Work out the finished part from the listing and answer in its coordinate system (mm). A direction names the side the tool comes from. Give positions to 0.01 mm unless a question says otherwise; leave off trailing zeros. Write each loop counter-clockwise with the first axis right and the second up, starting at its lowest first coordinate (ties: lowest second). Pieces come first, ordered by that corner, then holes.
1) A tool of negligible diameter and unlimited length cuts with its end or side. For faces 5 (the face through (-472.6, -3, 36)), 6 (the face through (254, -63.5, -138)), 7 (the face through (-242, 145, -38.1)), 8 (the face through (228.6, -76, -138)), 9 (the face through (254, 215.9, -138)), from which of +Z, -Z, +X, -X, +Y, -Y can it reach the whole face along a straight path? Write none if from no direction.
2) Find section A-A (y = 139.7). Determine the outline of the cut face in (x, z), plus the area to 3 significant figures.
3) Given pin 1 Ø3 at (x, y) = (-297.5, 79) entering from -Z; pin 2 Ø12.5 at (y, z) = (-71, -126) entering from +X; pin 3 Ø5 at (y, z) = (139, 181) entering from -X, each flat-ended and moving along its own axis, determine where each tip first touches the part or whether it passes through.
4) Straight lines are drawn through the part: probe 1 along Y at (x, z) = (-254, -21); probe 2 along Y at (x, z) = (-254, 5); probe 3 along Z at (x, y) = (-134, 181). For each, find the intervals that lie inside material, in ascending order.
5) Find section C-C (x = -157.5). Determine the outline of the cut face in (y, z), plus the area to 3 significant figures.
6) Determine the mould class of faces 1 (the face through (228.6, 76, -138)), 2 (the face through (-437.886, 3.815, -25.756)), 3 (the face through (254, 203, -228.6)), 4 (the face through (192.93, -20, 220.54)) for opening direction X: pulls with the +X half, pulls with the -X half, needs draft (parallel to the pull), parting line crosses it, or undercut.
7) Find section D-D (y = -34). Determine the outline of the cut face in (x, z).
8) Find section B-B (z = -61). Determine the outline of the cut face in (x, y), plus the area to 3 significant figures.
```python
from build123d import *

# Parameters (mm, degrees)
SKETCH1_W                = 965.2
SKETCH1_H                = 508
BOSS_EXTRUDE1_DEPTH      = 50.8
SKETCH3_W                = 50.8
SKETCH3_H                = 25.4
BOSS_EXTRUDE2_DEPTH      = 177.8
CUT_EXTRUDE2_DEPTH       = 592.334693723
CUT_EXTRUDE2_DEPTH_BACK  = 592.334693723
SKETCH4_R                = 12.7
BOSS_EXTRUDE3_DEPTH      = 254
BOSS_EXTRUDE3_DEPTH_BACK = 254
BOSS_EXTRUDE4_DEPTH      = 12.7
BOSS_EXTRUDE5_START      = -508
BOSS_EXTRUDE5_DEPTH      = 12.7
CUT_EXTRUDE3_DEPTH       = 592.556393084
CUT_EXTRUDE3_DEPTH_BACK  = 592.556393084
SKETCH2_R                = 12.7
CUT_EXTRUDE4_START       = -50.8
SKETCH12_R               = 25.4
SKETCH12_R_2             = 12.7
CUT_EXTRUDE4_DEPTH       = 12.7
SKETCH13_R               = 12.7
CUT_EXTRUDE5_DEPTH       = 25.4
CUT_EXTRUDE6_START       = -2.7
SKETCH14_R               = 25.4
SKETCH14_R_2             = 12.7
CUT_EXTRUDE6_DEPTH       = 12.7
CUT_EXTRUDE7_DEPTH       = 10
CUT_EXTRUDE7_DEPTH_BACK  = 592.556393084
SKETCH15_R               = 12.7
SKETCH2_4_R              = 12.7
BOSS_EXTRUDE6_DEPTH      = 150
CUT_EXTRUDE8_REACH       = 714.022
SKETCH16_R               = 4.5
CUT_EXTRUDE9_REACH       = 823.718
SKETCH17_W               = 300
SKETCH17_H               = 450


with BuildPart() as part:
    # Sketch1 → Boss-Extrude1 (new body)
    with BuildSketch(Plane.XY):
        Rectangle(SKETCH1_W, SKETCH1_H)
    extrude(amount=-BOSS_EXTRUDE1_DEPTH)

    # Sketch3 → Boss-Extrude2 (add)
    with BuildSketch(Plane(origin=(0, 0, -50.8), x_dir=(-1, 0, 0), z_dir=(0, 0, -1))):
        with Locations((-254, 203.2)):
            Rectangle(SKETCH3_W, SKETCH3_H)
        with Locations((-254, 76.2)):
            Rectangle(SKETCH3_W, SKETCH3_H)
        with Locations((-254, -76.2)):
            Rectangle(SKETCH3_W, SKETCH3_H)
        with Locations((-254, -203.2)):
            Rectangle(SKETCH3_W, SKETCH3_H)
    extrude(amount=BOSS_EXTRUDE2_DEPTH)

    # Sketch4 → Cut-Extrude2 (cut, two sides: drawn at the far end of the back side and taken through both)
    with BuildSketch(Plane(origin=(0, 0, 0), x_dir=(1, 0, 0), z_dir=(0, 1, 0)).offset(-CUT_EXTRUDE2_DEPTH_BACK)):
        with Locations(Location((254, 190.5, 0), (0, 0, 270))):
            Circle(SKETCH4_R)
    extrude(amount=CUT_EXTRUDE2_DEPTH + CUT_EXTRUDE2_DEPTH_BACK, mode=Mode.SUBTRACT)

    # Sketch10 → Boss-Extrude3 (add, two sides: drawn at the far end of the back side and taken through both)
    with BuildSketch(Plane(origin=(0, 0, 0), x_dir=(1, 0, 0), z_dir=(0, 1, 0)).offset(-BOSS_EXTRUDE3_DEPTH_BACK)):
        Polygon((482.6, 0), (-482.6, 0), (-482.6, -66.924314291), (-176.649889789, -229.172874046), (0, -229.172874046), (176.649889789, -229.172874046), (482.6, -66.924314291), align=None)
        Polygon((-472.6, -60.908279697), (-472.6, -10), (472.6, -10), (472.6, -60.908279697), (174.162404273, -219.172874046), (0, -219.172874046), (-174.162404273, -219.172874046), align=None, mode=Mode.SUBTRACT)
    extrude(amount=BOSS_EXTRUDE3_DEPTH + BOSS_EXTRUDE3_DEPTH_BACK)

    # Sketch11 → Boss-Extrude4 (add)
    with BuildSketch(Plane.XZ.offset(254)):
        Polygon((-472.6, 10), (-472.6, 60.908279697), (-174.162404273, 219.172874046), (174.162404273, 219.172874046), (472.6, 60.908279697), (472.6, 10), align=None)
    extrude(amount=-BOSS_EXTRUDE4_DEPTH)

    # Sketch11<2> → Boss-Extrude5 (add)
    with BuildSketch(Plane.XZ.offset(254).offset(BOSS_EXTRUDE5_START)):
        Polygon((-472.6, 10), (-472.6, 60.908279697), (-174.162404273, 219.172874046), (174.162404273, 219.172874046), (472.6, 60.908279697), (472.6, 10), align=None)
    extrude(amount=BOSS_EXTRUDE5_DEPTH)

    # Sketch2 → Cut-Extrude3 (cut, two sides: drawn at the far end of the back side and taken through both)
    with BuildSketch(Plane.XY.offset(-CUT_EXTRUDE3_DEPTH_BACK)):
        with Locations((-450, 0)):
            Circle(SKETCH2_R)
    extrude(amount=CUT_EXTRUDE3_DEPTH + CUT_EXTRUDE3_DEPTH_BACK, mode=Mode.SUBTRACT)

    # Sketch12 → Cut-Extrude4 (cut)
    # profile 1 of 2: a face of its own
    with BuildSketch(Plane.XY.offset(CUT_EXTRUDE4_START)):
        with Locations(Location((-254, 139.7, 0), (0, 0, 180))):
            Circle(SKETCH12_R)
        with Locations(Location((-254, 139.7, 0), (0, 0, 180))):
            Circle(SKETCH12_R_2, mode=Mode.SUBTRACT)
    # profile 2 of 2: a face of its own
    with BuildSketch(Plane.XY.offset(CUT_EXTRUDE4_START)):
        with Locations(Location((-254, -139.7, 0), (0, 0, 180))):
            Circle(SKETCH12_R)
        with Locations(Location((-254, -139.7, 0), (0, 0, 180))):
            Circle(SKETCH12_R_2, mode=Mode.SUBTRACT)
    extrude(amount=CUT_EXTRUDE4_DEPTH, mode=Mode.SUBTRACT)

    # Sketch13 → Cut-Extrude5 (cut)
    with BuildSketch(Plane(origin=(0, 0, -50.8), x_dir=(-1, 0, 0), z_dir=(0, 0, -1))):
        with Locations((254, 139.7)):
            Circle(SKETCH13_R)
        with Locations((254, -139.7)):
            Circle(SKETCH13_R)
    extrude(amount=-CUT_EXTRUDE5_DEPTH, mode=Mode.SUBTRACT)

    # Sketch14 → Cut-Extrude6 (cut)
    # profile 1 of 2: a face of its own
    with BuildSketch(Plane.XY.offset(CUT_EXTRUDE6_START)):
        with Locations(Location((-254, 139.7, 0), (0, 0, 180))):
            Circle(SKETCH14_R)
        with Locations(Location((-254, 139.7, 0), (0, 0, 180))):
            Circle(SKETCH14_R_2, mode=Mode.SUBTRACT)
    # profile 2 of 2: a face of its own
    with BuildSketch(Plane.XY.offset(CUT_EXTRUDE6_START)):
        with Locations(Location((-254, -139.7, 0), (0, 0, 180))):
            Circle(SKETCH14_R)
        with Locations(Location((-254, -139.7, 0), (0, 0, 180))):
            Circle(SKETCH14_R_2, mode=Mode.SUBTRACT)
    extrude(amount=CUT_EXTRUDE6_DEPTH, mode=Mode.SUBTRACT)

    # Sketch15 → Cut-Extrude7 (cut, two sides: drawn at the far end of the back side and taken through both)
    with BuildSketch(Plane.XY.offset(-CUT_EXTRUDE7_DEPTH_BACK)):
        with Locations(Location((-254, -139.7, 0), (0, 0, 180))):
            Circle(SKETCH15_R)
        with Locations(Location((-254, 139.7, 0), (0, 0, 180))):
            Circle(SKETCH15_R)
    extrude(amount=CUT_EXTRUDE7_DEPTH + CUT_EXTRUDE7_DEPTH_BACK, mode=Mode.SUBTRACT)

    # Sketch2<4> → Boss-Extrude6 (add)
    with BuildSketch(Plane.XY):
        with Locations((-450, 0)):
            Circle(SKETCH2_4_R)
    extrude(amount=BOSS_EXTRUDE6_DEPTH)

    # Sketch16 → Cut-Extrude8 (cut, up to next)
    with BuildSketch(Plane.XY.offset(229.172874046), mode=Mode.PRIVATE) as cut_extrude8_sk1:
        with Locations((-66, 0)):
            Circle(SKETCH16_R)
    cut_extrude8_tool1 = extrude(cut_extrude8_sk1.sketch, amount=-CUT_EXTRUDE8_REACH, mode=Mode.PRIVATE) & part.part
    # Sketch16 → Cut-Extrude8 (cut, up to next)
    with BuildSketch(Plane.XY.offset(229.172874046), mode=Mode.PRIVATE) as cut_extrude8_sk2:
        with Locations((0, 66)):
            Circle(SKETCH16_R)
    cut_extrude8_tool2 = extrude(cut_extrude8_sk2.sketch, amount=-CUT_EXTRUDE8_REACH, mode=Mode.PRIVATE) & part.part
    # Sketch16 → Cut-Extrude8 (cut, up to next)
    with BuildSketch(Plane.XY.offset(229.172874046), mode=Mode.PRIVATE) as cut_extrude8_sk3:
        with Locations((66, 0)):
            Circle(SKETCH16_R)
    cut_extrude8_tool3 = extrude(cut_extrude8_sk3.sketch, amount=-CUT_EXTRUDE8_REACH, mode=Mode.PRIVATE) & part.part
    # Sketch16 → Cut-Extrude8 (cut, up to next)
    with BuildSketch(Plane.XY.offset(229.172874046), mode=Mode.PRIVATE) as cut_extrude8_sk4:
        with Locations((0, -66)):
            Circle(SKETCH16_R)
    cut_extrude8_tool4 = extrude(cut_extrude8_sk4.sketch, amount=-CUT_EXTRUDE8_REACH, mode=Mode.PRIVATE) & part.part
    add(cut_extrude8_tool1.solids().sort_by_distance((-66, 0, 229.172874))[0], mode=Mode.SUBTRACT)
    add(cut_extrude8_tool2.solids().sort_by_distance((0, 66, 229.172874))[0], mode=Mode.SUBTRACT)
    add(cut_extrude8_tool3.solids().sort_by_distance((66, 0, 229.172874))[0], mode=Mode.SUBTRACT)
    add(cut_extrude8_tool4.solids().sort_by_distance((0, -66, 229.172874))[0], mode=Mode.SUBTRACT)

    # Sketch17 → Cut-Extrude9 (cut, up to next)
    with BuildSketch(Plane(origin=(133.630964067, 0, 251.986262594), x_dir=(0.8834593660439969, 0, -0.4685077892086097), z_dir=(0.4685077892086097, 0, 0.8834593660439969)), mode=Mode.PRIVATE) as cut_extrude9_sk1:
        with Locations((217.872449791, 0)):
            Rectangle(SKETCH17_W, SKETCH17_H)
    cut_extrude9_tool1 = extrude(cut_extrude9_sk1.sketch, amount=-CUT_EXTRUDE9_REACH, mode=Mode.PRIVATE) & part.part
    add(cut_extrude9_tool1.solids().sort_by_distance((326.11242, 0, 149.911323))[0], mode=Mode.SUBTRACT)


solid = part.part
```
Results:
1. face 5: none
1. face 6: -Z, +X, -X
1. face 7: -Z
1. face 8: -Z, -X, +Y, -Y
1. face 9: -Z, +X, -X, +Y
2. outline: (-482.6, -50.8) - (-279.4, -50.8) - (-279.4, -38.1) - (-266.7, -38.1) - (-266.7, -2.7) - (-279.4, -2.7) - (-279.4, 10) - (-472.6, 10) - (-472.6, 60.91) - (-174.16, 219.17) - (174.16, 219.17) - (188.91, 211.35) - (193.59, 220.19) - (176.65, 229.17) - (-176.65, 229.17) - (-482.6, 66.92) - close; (-241.3, -38.1) - (-228.6, -38.1) - (-228.6, -50.8) - (482.6, -50.8) - (482.6, 66.92) - (458.63, 79.64) - (453.95, 70.8) - (472.6, 60.91) - (472.6, 10) - (-228.6, 10) - (-228.6, -2.7) - (-241.3, -2.7) - close
2. area: 64,900 mm2
3. pin 1: stops at z = -50.8
3. pin 2: stops at x = 279.4
3. pin 3: stops at x = -272.2
4. probe 1: y = -254 to -152.4, -127 to 127, 152.4 to 254
4. probe 2: y = -254 to -165.1, -114.3 to 114.3, 165.1 to 254
4. probe 3: z = -50.8 to 10, 219.17 to 229.17
5. outline: (-254, -50.8) - (254, -50.8) - (254, 229.17) - (-254, 229.17) - close; hole (-241.3, 10) - (241.3, 10) - (241.3, 219.17) - (-241.3, 219.17) - close
5. area: 41,300 mm2
6. face 1: pulls with the -X half
6. face 2: undercut
6. face 3: needs draft
6. face 4: pulls with the +X half
7. outline: (-482.6, -50.8) - (482.6, -50.8) - (482.6, 66.92) - (458.63, 79.64) - (453.95, 70.8) - (472.6, 60.91) - (472.6, 10) - (-472.6, 10) - (-472.6, 60.91) - (-174.16, 219.17) - (174.16, 219.17) - (188.91, 211.35) - (193.59, 220.19) - (176.65, 229.17) - (-176.65, 229.17) - (-482.6, 66.92) - close
8. outline: (228.6, -215.9) - (279.4, -215.9) - (279.4, -190.5) - (228.6, -190.5) - close; (228.6, -88.9) - (279.4, -88.9) - (279.4, -63.5) - (228.6, -63.5) - close; (228.6, 63.5) - (279.4, 63.5) - (279.4, 88.9) - (228.6, 88.9) - close; (228.6, 190.5) - (279.4, 190.5) - (279.4, 215.9) - (228.6, 215.9) - close
8. area: 5,160 mm2
